CAD build for the part. Positions are in the model's coordinates, mm. Give positions to 0.01 mm unless a question says otherwise; leave off trailing zeros. Loops run counter-clockwise (first coordinate to the right, second up) from the corner with the lowest first, then second, coordinate; pieces in that order, holes last. Notation, with made-up numbers: M 33.25,48.5 L 90.25,48.5 A33 cw 90.25,80.5 Z; hole C 37.5,71 d11. An arc over 180 degrees is marked long. Answer as CSV lines item,"result".
from build123d import *

# Parameters (mm, degrees)
BOSS_EXTRUDE2_DEPTH = 8
SKETCH2_R           = 1.5
CUT_EXTRUDE1_DEPTH  = 211.61424354


with BuildPart() as part:
    # Sketch1 → Boss-Extrude2 (new body)
    with BuildSketch(Plane(origin=(0, 0, 0), x_dir=(1, 0, 0), z_dir=(0, 1, 0))):
        Polygon((94.000414938, -26.09989937), (30.400414938, 84.058531992), (-96.799585062, 84.058531992), (-160.399585062, -26.09989937), (-96.799585062, -136.258330731), (30.400414938, -136.258330731), align=None)
    extrude(amount=BOSS_EXTRUDE2_DEPTH)

    # Sketch2 → Cut-Extrude1 (cut, through all)
    with BuildSketch(Plane(origin=(0, 8, 0), x_dir=(1, 0, 0), z_dir=(0, 1, 0))):
        with Locations(Location((17.780367394, -130.408330731, 0), (0, 0, 270))):
            Circle(SKETCH2_R)
        with Locations(Location((-84.179537519, -130.408330731, 0), (0, 0, 270))):
            Circle(SKETCH2_R)
        with Locations(Location((-84.221416865, -114.108384531, 0), (0, 0, 270))):
            Circle(SKETCH2_R)
        with Locations(Location((17.566684484, -114.109731417, 0), (0, 0, 270))):
            Circle(SKETCH2_R)
        with Locations(Location((82.624142554, -18.0956176, 0), (0, 0, 270))):
            Circle(SKETCH2_R)
        with Locations(Location((68.507928472, -26.2456176, 0), (0, 0, 270))):
            Circle(SKETCH2_R)
        with Locations(Location((31.676359033, 70.148531992, 0), (0, 0, 270))):
            Circle(SKETCH2_R)
        with Locations(Location((17.560144951, 61.998531992, 0), (0, 0, 270))):
            Circle(SKETCH2_R)
        with Locations(Location((-98.075529157, 70.148531992, 0), (0, 0, 270))):
            Circle(SKETCH2_R)
        with Locations(Location((-83.959315075, 61.998531992, 0), (0, 0, 270))):
            Circle(SKETCH2_R)
        with Locations(Location((-149.023312678, -18.0956176, 0), (0, 0, 270))):
            Circle(SKETCH2_R)
        with Locations(Location((-134.907098597, -26.2456176, 0), (0, 0, 270))):
            Circle(SKETCH2_R)
    extrude(amount=-CUT_EXTRUDE1_DEPTH, mode=Mode.SUBTRACT)


solid = part.part
1) Band-saw the part on B-B on z = -23. Give the cut face in (x, y).
Answer below:
outline,"M -132.05,0 L 65.65,0 L 65.65,8 L -132.05,8 Z"
2) Band-saw the part on C-C on x = -144. Give the cut face in (y, z), and give its area (3 significant figures).
Answer below:
outline,"M 0,-2.31 L 8,-2.31 L 8,54.5 L 0,54.5 Z"
area,"454 mm^2"
3) Band-saw the part on A-A on y = 4. Give the number of separate pieces and of enclosed holes in the cut face, and give its area (3 significant figures).
Answer below:
separate pieces,"1"
enclosed holes,"12"
area,"42,000 mm^2"
4) Flat gauge pins, fed straight in: pin 1 (1.5 mm diameter, centred on x = 47, y = 6.5, fed in from +Z); pin 2 (3 mm diameter, centred on y = 6, z = 65.5, fed in from -X); pin 3 (2 mm diameter, centred on y = 2.5, z = 23.5, fed in from +X). Where does each tip first touch, or does it go through?
Answer below:
pin 1,"stops at z = 108.81"
pin 2,"stops at x = -138.52"
pin 3,"stops at x = 93.08"
5) Drill centre lines: line 1 (Z direction, x = -113, y = 4.25); line 2 (X direction, y = 3, z = 34.5); line 3 (X direction, y = 2, z = 0). Where is each one in solid material? Low to high. Write a range as from..to.
Answer below:
line 1,"z = -56..108.2"
line 2,"x = -155.55..89.15"
line 3,"x = -145.33..78.93"
